```python
from build123d import *

# Parameters (mm, degrees)
SKICA1_W                 = 101.6
SKICA1_H                 = 147
P_IDAT_VYSUNUT_M1_DEPTH  = 26.1
SKICA3_W                 = 85.062789824
SKICA3_H                 = 9.622095786
ODEBRAT_VYSUNUT_M2_DEPTH = 9
SKICA2_R                 = 1.7526
ODEBRAT_VYSUNUT_M1_DEPTH = 5
SKICA4_R                 = 1.7526
ODEBRAT_VYSUNUT_M3_DEPTH = 5


with BuildPart() as part:
    # Skica1 → Přidat vysunutím1 (new body)
    with BuildSketch(Plane(origin=(0, 0, 0), x_dir=(1, 0, 0), z_dir=(0, 1, 0))):
        Rectangle(SKICA1_W, SKICA1_H)
    extrude(amount=P_IDAT_VYSUNUT_M1_DEPTH)

    # Skica3 → Odebrat vysunutím2 (cut)
    with BuildSketch(Plane.XY.offset(73.5)):
        with Locations((3.263182855, 8.448501867)):
            Rectangle(SKICA3_W, SKICA3_H)
    extrude(amount=-ODEBRAT_VYSUNUT_M2_DEPTH, mode=Mode.SUBTRACT)

    # Skica2 → Odebrat vysunutím1 (cut)
    with BuildSketch(Plane.XZ):
        with Locations(Location((-47.62, 32.22, 0), (0, 0, 270))):
            Circle(SKICA2_R)
        with Locations(Location((-47.62, -12.23, 0), (0, 0, 270))):
            Circle(SKICA2_R)
        with Locations(Location((-47.62, -43.98, 0), (0, 0, 270))):
            Circle(SKICA2_R)
    odebrat_vysunut_m1 = extrude(amount=-ODEBRAT_VYSUNUT_M1_DEPTH, mode=Mode.SUBTRACT)

    # Skica4 → Odebrat vysunutím3 (cut)
    with BuildSketch(Plane.ZY.offset(50.8)):
        with Locations((45, 4.567395648)):
            Circle(SKICA4_R)
        with Locations((-56.6, 4.567395648)):
            Circle(SKICA4_R)
    odebrat_vysunut_m3 = extrude(amount=-ODEBRAT_VYSUNUT_M3_DEPTH, mode=Mode.SUBTRACT)

    # Zrcadlit1: Odebrat vysunutím1, Odebrat vysunutím3 across plane
    add(odebrat_vysunut_m1.mirror(Plane(origin=(0, 0, 0), x_dir=(0, 0, 1), z_dir=(1, 0, 0))), mode=Mode.SUBTRACT)
    add(odebrat_vysunut_m3.mirror(Plane(origin=(0, 0, 0), x_dir=(0, 0, 1), z_dir=(1, 0, 0))), mode=Mode.SUBTRACT)


solid = part.part
```
Build history of the part. All positions in model axes, mm. A direction names the side the tool comes from. Give positions to 0.01 mm unless a question says otherwise; leave off trailing zeros. Order: outer loops, then holes, each group sorted by start corner. A loop starts at its lowest first (then second) coordinate and runs counter-clockwise, first axis right, second up. Notation, with made-up numbers: M 21.25,32.5 L 61.25,32.5 A24 cw 61.25,50.5 Z; hole C 80,6.5 d11. An arc over 180 degrees is marked long. Return JSON: item names as keys, results as strings.
Q1. Two-plate mould, pull along Z, no slides. Class faces 4 (the face through (-39.268, 8, 69)), 5 (the face through (3, 9, 64.5)), 6 (the face through (45.8, 5, 45)): pulls with the +Z half, pulls with the -Z half, needs draft (parallel to the pull), parting line crosses it, or undercut.
Answer list:
{"face 4": "needs draft", "face 5": "pulls with the +Z half", "face 6": "undercut"}
Q2. Band-saw the part on A-A (x = 44). Give the cut face in (y, z).
Answer list:
{"outline": "M 0,-73.5 L 26.1,-73.5 L 26.1,73.5 L 13.26,73.5 L 13.26,64.5 L 3.64,64.5 L 3.64,73.5 L 0,73.5 Z"}
Q3. Flat gauge pins, fed straight in: pin 1 (5.5 mm diameter, centred on x = -47.62, z = -43.98, fed in from -Y); pin 2 (3 mm diameter, centred on x = 47.62, z = -12.23, fed in from -Y); pin 3 (3 mm diameter, centred on x = -11, y = 5.5, fed in from +Z); pin 4 (3 mm diameter, centred on y = 4.57, z = 45, fed in from +X). Where does each tip first touch, or does it go through?
Answer list:
{"pin 1": "stops at y = 0", "pin 2": "stops at y = 5", "pin 3": "stops at z = 64.5", "pin 4": "stops at x = 45.8"}
Q4. 3-axis set-ups, long thin cutter, end or side, ignore diameter. For faces 1 (the face through (-45.8, 5, 45)), 2 (the face through (-49.175, 2.465, -44.789)), 3 (the face through (3, 13.26, 69)): which of +Z, -Z, +X, -X, +Y, -Y reach the whole face in a straight line?
Answer list:
{"face 1": "-X", "face 2": "-Y", "face 3": "+Z"}
Q5. Band-saw the part on B-B (y = 8.75). Give the cut face in (x, z), then the cut area to 3 significant figures.
Answer list:
{"outline": "M -50.8,-73.5 L 50.8,-73.5 L 50.8,73.5 L 45.79,73.5 L 45.79,64.5 L -39.27,64.5 L -39.27,73.5 L -50.8,73.5 Z", "area": "14,200 mm^2"}
Q6. Wall check: probe 1 along X at (y, z) = (3.7, -12.23); probe 2 along Z at (x, y) = (47.62, 2.6); probe 3 along Y at (x, z) = (-48.45, 45). Give the ranges that are in metal, low to high. Write a range as from..to.
Answer list:
{"probe 1": "x = -50.8..-49.37, -45.87..45.87, 49.37..50.8", "probe 2": "z = -73.5..-45.73, -42.23..-13.98, -10.48..30.47, 33.97..73.5", "probe 3": "y = 0..2.81, 6.32..26.1"}
